Source: CAD feature listing. Evaluate the final solid. Frame: model axes, mm. Face numbers are marked on the shaded views. A direction names the side the tool comes from. Round coordinates to 2 decimals unless told otherwise and drop trailing zeros. Order: outer loops, then holes, each group sorted by start corner. A loop starts at its lowest first (then second) coordinate and runs counter-clockwise, first axis right, second up. Notation, with made-up numbers: (71.5, 9) -> (121.5, 9) arc R23 ccw to (121.5, 43) -> close; hole circle Ø2 at (-11, 84). An arc over 180 degrees is marked (long way). Write item = value, one per line. Start each with the question number.
(1) Reachability of the marked faces 1, 2 and 3 from +Z, -Z, +X, -X, +Y, -Y: full face, straight path, thin tool, end or side. Return the list, or none.
(2) Ray query, line 1 (Z direction, x = 0, y = 4.65); line 2 (X direction, y = 5.25, z = 2.75). Return the intervals inside material, ascending.
(3) Contact query for flat-ended pins moving along their axis: pin 1 Ø1 at (x, z) = (-6, 1.5) entering from +Y; pin 2 Ø0.7 at (y, z) = (5, -2) entering from -X; pin 3 Ø1.4 at (y, z) = (5.5, 3.5) entering from +X. Output: stop coordinate, or through.
(4) Cut plane C-C on z = 4.5. Return the cut outline in (x, y).
(5) Cut plane B-B on y = 4.75. Return the cut outline in (x, z), then the cut area to 3 significant figures.
(6) Cut plane D-D on x = -1.5. Return the cut outline in (y, z).
(7) Cut plane A-A on z = 0. Return the cut outline in (x, y), then the cut area to 3 significant figures.
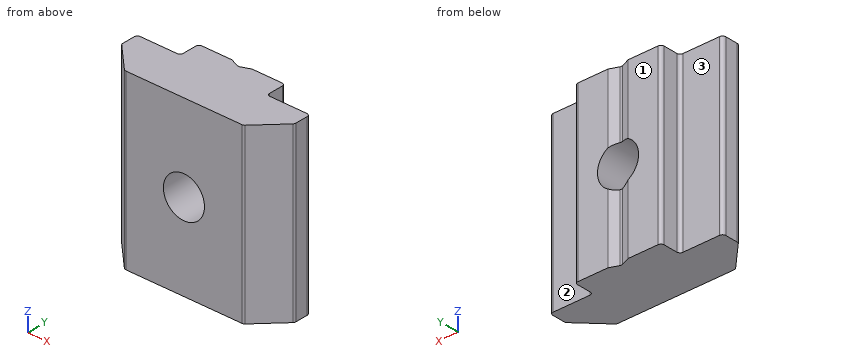
from build123d import *

# Parameters (mm, degrees)
BOSS_EXTRUDE1_DEPTH      = 8
BOSS_EXTRUDE1_DEPTH_BACK = 8
SKETCH9_R                = 1.9
CUT_EXTRUDE2_DEPTH       = 13.806248475
FILLET1_R                = 0.3


with BuildPart() as part:
    # Sketch4 → Boss-Extrude1 (new, two sides: drawn at the far end of the back side and taken through both)
    with BuildSketch(Plane.XY.offset(-BOSS_EXTRUDE1_DEPTH_BACK)):
        Polygon((-8, 4.1), (-8, 2.5), (-5.5, 0), (5.5, 0), (8, 2.5), (8, 4.1), (4, 4.1), (4, 6), (0.940533004, 6), (0, 5.62), (-0.940533004, 6), (-4, 6), (-4, 4.1), align=None)
    extrude(amount=BOSS_EXTRUDE1_DEPTH + BOSS_EXTRUDE1_DEPTH_BACK)

    # Sketch9 → Cut-Extrude2 (cut, through all)
    with BuildSketch(Plane(origin=(0, 0, 0), x_dir=(1, 0, 0), z_dir=(0, 1, 0))):
        with Locations(Location((0, 0, 0), (0, 0, 270))):
            Circle(SKETCH9_R)
    extrude(amount=CUT_EXTRUDE2_DEPTH, mode=Mode.SUBTRACT)

    # Fillet1
    # the kernel refuses this fillet: 0.3 mm, written as the material it adds along each edge
    with BuildSketch(Plane(origin=(-4, 4.1, 8), x_dir=(-1, 0, 0), z_dir=(0, 0, -1)), Plane(origin=(4, 4.1, -8), x_dir=(1, 0, 0), z_dir=(0, 0, 1))) as fillet1_piece_1:
        with BuildLine():
            CenterArc((FILLET1_R, FILLET1_R), FILLET1_R, 180, 90)
            Line((0, FILLET1_R), (0, 0))
            Line((0, 0), (FILLET1_R, 0))
        make_face()
    extrude(amount=16)
    with BuildSketch(Plane(origin=(0, 5.62, -8), x_dir=(0.927183854566788, 0.3746065934159107, 0), z_dir=(0, 0, 1))) as fillet1_piece_2_section:
        with BuildLine():
            CenterArc((FILLET1_R * 0.404026225835, FILLET1_R), FILLET1_R, 226, 44)
            Line((-FILLET1_R * 0.290632144624, FILLET1_R * 0.280660199661), (0, 0))
            Line((0, 0), (FILLET1_R * 0.404026225835, 0))
        make_face()
    fillet1_piece_2 = extrude(amount=6.403019669, mode=Mode.PRIVATE)
    fillet1_piece_2 = fillet1_piece_2 - Plane(origin=(0, 5.639105269, 0), x_dir=(0, 0, 1), z_dir=(0, -1, 0)) * Cylinder(1.9, 14, mode=Mode.PRIVATE)
    add(fillet1_piece_2)
    with BuildSketch(Plane(origin=(0, 5.62, 1.596980331), x_dir=(0.927183854566788, 0.3746065934159107, 0), z_dir=(0, 0, 1))) as fillet1_piece_3_section:
        with BuildLine():
            CenterArc((FILLET1_R * 0.404026225835, FILLET1_R), FILLET1_R, 226, 44)
            Line((-FILLET1_R * 0.290632144624, FILLET1_R * 0.280660199661), (0, 0))
            Line((0, 0), (FILLET1_R * 0.404026225835, 0))
        make_face()
    fillet1_piece_3 = extrude(amount=6.403019669, mode=Mode.PRIVATE)
    fillet1_piece_3 = fillet1_piece_3 - Plane(origin=(0, 5.639105269, 0), x_dir=(0, 0, 1), z_dir=(0, -1, 0)) * Cylinder(1.9, 14, mode=Mode.PRIVATE)
    add(fillet1_piece_3)
    # the kernel refuses this fillet: 0.3 mm, written as the material it takes off along each edge
    with BuildSketch(Plane(origin=(-4, 6, 8.75), x_dir=(1, 0, 0), z_dir=(0, 0, -1))) as fillet1_2_piece_1:
        with BuildLine():
            CenterArc((FILLET1_R, FILLET1_R), FILLET1_R, 180, 90)
            Line((0, FILLET1_R), (0, 0))
            Line((0, 0), (FILLET1_R, 0))
        make_face()
    extrude(amount=17.5, mode=Mode.SUBTRACT)
    with BuildSketch(Plane(origin=(-8, 4.1, 8.75), x_dir=(0, -1, 0), z_dir=(0, 0, -1)), Plane(origin=(8, 4.1, -8.75), x_dir=(0, -1, 0), z_dir=(0, 0, 1)), Plane(origin=(4, 6, -8.75), x_dir=(0, -1, 0), z_dir=(0, 0, 1))) as fillet1_2_piece_2:
        with BuildLine():
            CenterArc((FILLET1_R, -FILLET1_R), FILLET1_R, 90, 90)
            Line((0, -FILLET1_R), (0, 0))
            Line((0, 0), (FILLET1_R, 0))
        make_face()
    extrude(amount=17.5, mode=Mode.SUBTRACT)
    with BuildSketch(Plane(origin=(-8, 2.5, -8.310660172), x_dir=(0, 1, 0), z_dir=(0, 0, 1)), Plane(origin=(-5.5, 0, -8.310660172), x_dir=(-0.7071067811865439, 0.7071067811865512, 0), z_dir=(0, 0, 1)), Plane(origin=(5.5, 0, -8.310660172), x_dir=(-1, 0, 0), z_dir=(0, 0, 1)), Plane(origin=(8, 2.5, -8.310660172), x_dir=(-0.7071067811865492, -0.7071067811865457, 0), z_dir=(0, 0, 1))) as fillet1_2_piece_3:
        with BuildLine():
            CenterArc((FILLET1_R * 0.414213562373, -FILLET1_R), FILLET1_R, 90, 45)
            Line((-FILLET1_R * 0.292893218813, -FILLET1_R * 0.292893218813), (0, 0))
            Line((0, 0), (FILLET1_R * 0.414213562373, 0))
        make_face()
    extrude(amount=16.621320344, mode=Mode.SUBTRACT)


solid = part.part
Evaluation:
q1.face_1 = +Z, -Z, +X, -X, +Y
q1.face_2 = +Z, -Z, +X, +Y
q1.face_3 = +Z, -Z, -X, +Y
q2.line_1 = -8 to -1.9, 1.9 to 8
q2.line_2 = -4 to 4
q3.pin_1 = 4.1
q3.pin_2 = -4
q3.pin_3 = 4
q4.outline = (-8, 2.62) arc R0.3 ccw to (-7.91, 2.41) -> (-5.59, 0.09) arc R0.3 ccw to (-5.38, 0) -> (5.38, 0) arc R0.3 ccw to (5.59, 0.09) -> (7.91, 2.41) arc R0.3 ccw to (8, 2.62) -> (8, 3.8) arc R0.3 ccw to (7.7, 4.1) -> (4.3, 4.1) arc R0.3 cw to (4, 4.4) -> (4, 5.7) arc R0.3 ccw to (3.7, 6) -> (0.94, 6) -> (0.11, 5.67) arc R0.3 cw to (-0.11, 5.67) -> (-0.94, 6) -> (-3.7, 6) arc R0.3 ccw to (-4, 5.7) -> (-4, 4.4) arc R0.3 cw to (-4.3, 4.1) -> (-7.7, 4.1) arc R0.3 ccw to (-8, 3.8) -> close
q5.outline = (-4, -8) -> (4, -8) -> (4, 8) -> (-4, 8) -> close; hole circle Ø3.8 at (0, 0)
q5.area = 117 mm^2
q6.outline = (0, -8) -> (6, -8) -> (6, -1.17) -> (0, -1.17) -> close; (0, 1.17) -> (6, 1.17) -> (6, 8) -> (0, 8) -> close
q7.outline = (-8, 2.62) arc R0.3 ccw to (-7.91, 2.41) -> (-5.59, 0.09) arc R0.3 ccw to (-5.38, 0) -> (-1.9, 0) -> (-1.9, 6) -> (-3.7, 6) arc R0.3 ccw to (-4, 5.7) -> (-4, 4.4) arc R0.3 cw to (-4.3, 4.1) -> (-7.7, 4.1) arc R0.3 ccw to (-8, 3.8) -> close; (1.9, 0) -> (5.38, 0) arc R0.3 ccw to (5.59, 0.09) -> (7.91, 2.41) arc R0.3 ccw to (8, 2.62) -> (8, 3.8) arc R0.3 ccw to (7.7, 4.1) -> (4.3, 4.1) arc R0.3 cw to (4, 4.4) -> (4, 5.7) arc R0.3 ccw to (3.7, 6) -> (1.9, 6) -> close
q7.area = 51.7 mm^2
